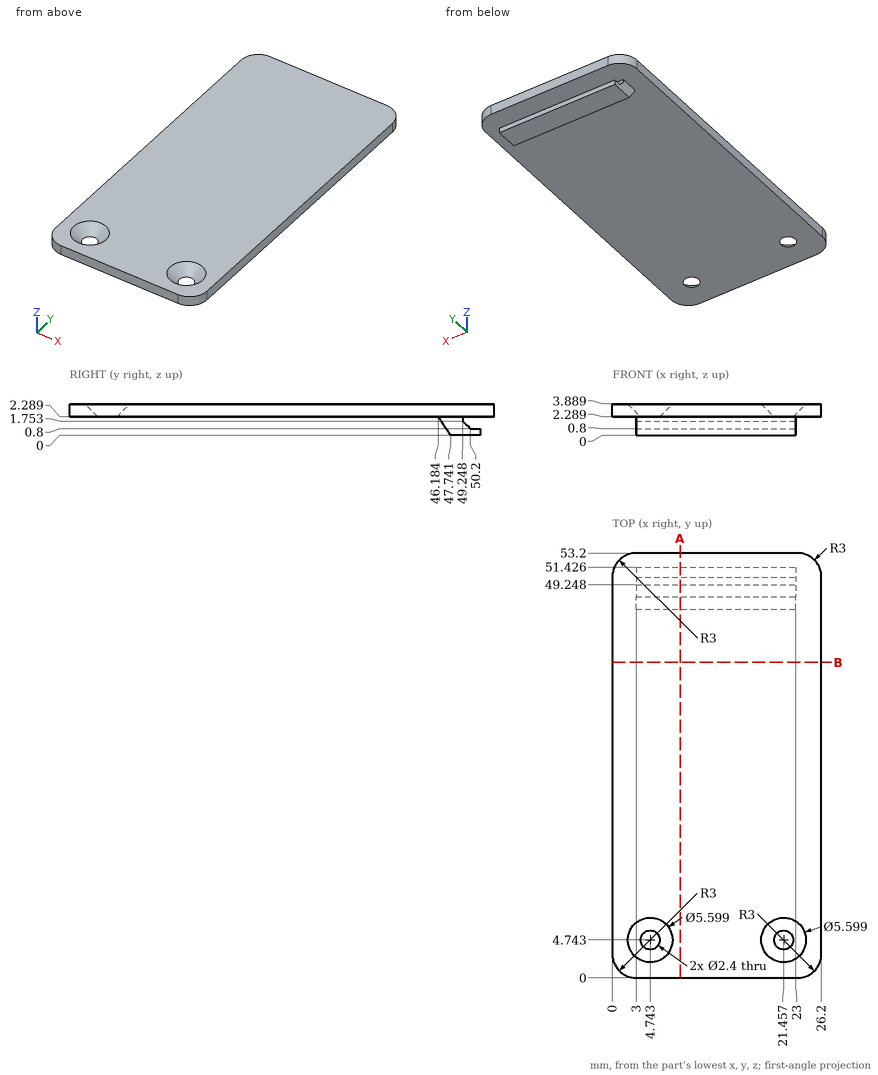
Here's the drawing with two shaded views (mm, measured from the low corner). I have some questions. Coordinates: 2 decimals unless noted, no trailing zeros. Order: outer loops, then holes, each group sorted by start corner. A loop starts at its lowest first (then second) coordinate and runs counter-clockwise, first axis right, second up. Notation, with made-up numbers: (-13.75, 11) - (36.25, 11) arc R5 ccw to (36.25, 17) - close; hole circle Ø11 at (1.25, 29.25). An arc over 180 degrees is marked (long way). Answer in a Markdown table with one row per item. Add a question column.
(1) I need wall thicknesses on L1, parallel to Z at x = 20.75, y = 26.5; L2, parallel to X at y = 49, z = 0.95; L3, parallel to Y at x = 21.75, z = 1.25. Which ranges of each line are inside material? Lowest first, please.
(2) If we section it at A-A, the plane x = 8.5: Please give me the cut outline in (y, z) (1 decimal).
(3) If we section it at B-B, the plane y = 39.5: Please give me the cut outline in (x, z).
(4) Will these pins go through, and if not, where does the flat tip stop? pin 1 (3 mm diameter, centred on x = 12, y = 19.5, fed in from -Z); pin 2 (1.8 mm diameter, centred on y = 48, z = 1, fed in from +X).
Results are:
| question | item | result |
|---|---|---|
| 1 | L1 | z = 2.29 to 3.89 |
| 1 | L2 | x = 3 to 23 |
| 1 | L3 | y = 46.89 to 49.75 |
| 2 | outline | (0, 2.3) - (46.2, 2.3) - (47.7, 0) - (51.4, 0) - (51.4, 0.8) - (50.2, 0.8) - (49.2, 1.8) - (49.2, 2.3) - (53.2, 2.3) - (53.2, 3.9) - (0, 3.9) - close |
| 3 | outline | (0, 2.29) - (26.2, 2.29) - (26.2, 3.89) - (0, 3.89) - close |
| 4 | pin 1 | stops at z = 2.29 |
| 4 | pin 2 | stops at x = 23 |
